from build123d import *


with BuildPart() as part:
    # Sketch2 → Revolve1 (revolve)
    with BuildSketch(Plane.XY):
        with BuildLine():
            ThreePointArc((0, 2.375), (0.992680215, 3.754414901), (2.37, 4.75))
            Line((2.37, 4.75), (2.75, 4.75))
            Line((2.75, 4.75), (2.75, 2.5))
            Line((2.75, 2.5), (17.75, 2.5))
            Line((17.75, 2.5), (17.75, 4.75))
            Line((17.75, 4.75), (18.13, 4.75))
            ThreePointArc((18.13, 4.75), (19.507319785, 3.754414901), (20.5, 2.375))
            Line((20.5, 2.375), (20.5, 0))
            Line((20.5, 0), (0, 0))
            Line((0, 0), (0, 2.375))
        make_face()
    revolve(axis=Axis((-1.178114582, 0, 0), (1, 0, 0)))


solid = part.part
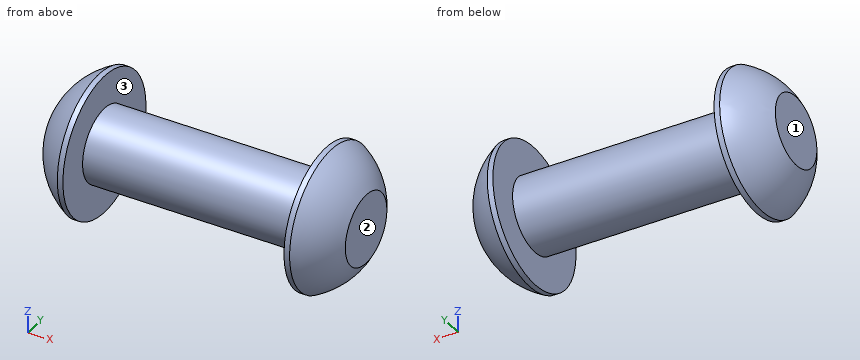
Source: CAD feature listing. Evaluate the final solid. Frame: model axes, mm. Face numbers are marked on the shaded views. Coordinates: 2 decimals unless noted, no trailing zeros. Write each loop counter-clockwise with the first axis right and the second up, starting at its lowest first coordinate (ties: lowest second). Pieces come first, ordered by that corner, then holes. Notation, with made-up numbers: M 84.5,53 L 111.5,53 A27 ccw 111.5,75 Z; hole C -17.75,59.5 d5. An arc over 180 degrees is marked long. Use a Markdown table: item, result.
1) Section B-B, the plane z = -3.75. Output: boundary loops of the cut face in (x, y).
Conclusion:
| item | result |
|---|---|
| outline | M 2.37,-2.92 L 2.75,-2.92 L 2.75,2.92 L 2.37,2.92 A3.77 ccw Z; M 17.75,-2.92 L 18.13,-2.92 A3.77 ccw 18.13,2.92 L 17.75,2.92 Z |
2) First-contact query: pin 1 Ø1 at (x, y) = (16.5, -1.5) entering from -Z; pin 2 Ø1 at (x, y) = (18, -2) entering from -Z; pin 3 Ø2 at (x, y) = (7.5, -3) entering from +Z. Flat tips, straight axial feed; report the tip coordinate or a pass-through.
Conclusion:
| item | result |
|---|---|
| pin 1 | stops at z = -2.29 |
| pin 2 | stops at z = -4.51 |
| pin 3 | stops at z = 1.5 |
3) Section C-C, the plane y = -3.5. Output: boundary loops of the cut face in (x, z), then the cut area to 3 significant figures.
Conclusion:
| item | result |
|---|---|
| outline | M 2.37,-3.21 L 2.75,-3.21 L 2.75,3.21 L 2.37,3.21 A4 ccw Z; M 17.75,-3.21 L 18.13,-3.21 A4 ccw 18.13,3.21 L 17.75,3.21 Z |
| area | 19.4 mm^2 |
4) Ray query, L1, parallel to X at y = -3.25, z = 1; L2, parallel to X at y = 4, z = 2; L3, parallel to Z at x = 6.75, y = 1. Return the intervals inside material, ascending.
Conclusion:
| item | result |
|---|---|
| L1 | x = 0.67 to 2.75, 17.75 to 19.83 |
| L2 | x = 1.88 to 2.75, 17.75 to 18.62 |
| L3 | z = -2.29 to 2.29 |
5) Section A-A, the plane y = 0. Output: boundary loops of the cut face in (x, z) (3 decimals).
Conclusion:
| item | result |
|---|---|
| outline | M 0,-2.375 A5.315 ccw 2.37,-4.75 L 2.75,-4.75 L 2.75,-2.5 L 17.75,-2.5 L 17.75,-4.75 L 18.13,-4.75 A5.315 ccw 20.5,-2.375 L 20.5,2.375 A5.315 ccw 18.13,4.75 L 17.75,4.75 L 17.75,2.5 L 2.75,2.5 L 2.75,4.75 L 2.37,4.75 A5.315 ccw 0,2.375 Z |
6) Mould query, pull axis X, two halves, no side actions, for the marked faces 1, 2 and 3. Classes: pulls with the +X half, pulls with the -X half, needs draft (parallel to the pull), parting line crosses it, or undercut.
Conclusion:
| item | result |
|---|---|
| face 1 | pulls with the -X half |
| face 2 | pulls with the +X half |
| face 3 | undercut |
